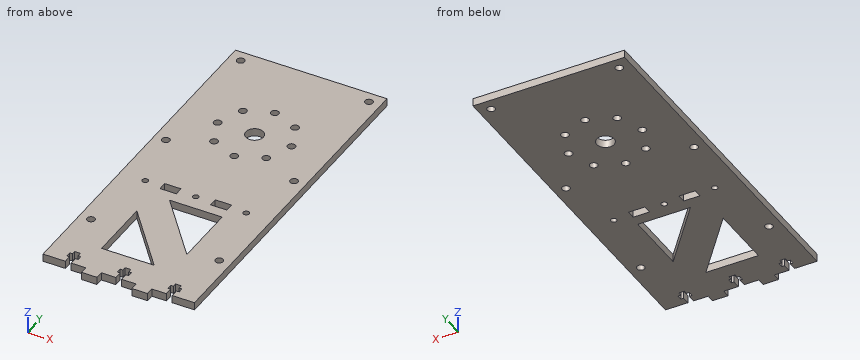
```python
from build123d import *

# Parameters (mm, degrees)
SKETCH_1_W          = 78
SKETCH_1_H          = 180
SKETCH_1_R          = 4.5
SKETCH_1_R_2        = 2
EXTRUDE_1_DEPTH     = 4
SKETCH_2_R          = 1.5
SKETCH_2_W          = 8.4
SKETCH_2_H          = 4.4
CUT_EXTRUDE_1_DEPTH = 4
SKETCH_6_W          = 8
SKETCH_6_H          = 8
EXTRUDE_2_DEPTH     = 4
SKETCH_7_R          = 2
CUT_EXTRUDE_2_DEPTH = 10


with BuildPart() as part:
    # 草图1 → 凸台-拉伸1 (new body)
    with BuildSketch(Plane.XY):
        with Locations((-4, -57.5)):
            Rectangle(SKETCH_1_W, SKETCH_1_H)
        with Locations((-4, -20.5)):
            Circle(SKETCH_1_R, mode=Mode.SUBTRACT)
        with Locations((15, -20.5)):
            Circle(SKETCH_1_R_2, mode=Mode.SUBTRACT)
        with Locations((9.435028843, -33.935028843)):
            Circle(SKETCH_1_R_2, mode=Mode.SUBTRACT)
        with Locations((-4, -39.5)):
            Circle(SKETCH_1_R_2, mode=Mode.SUBTRACT)
        with Locations((-17.435028843, -33.935028843)):
            Circle(SKETCH_1_R_2, mode=Mode.SUBTRACT)
        with Locations((-23, -20.5)):
            Circle(SKETCH_1_R_2, mode=Mode.SUBTRACT)
        with Locations((-17.435028843, -7.064971157)):
            Circle(SKETCH_1_R_2, mode=Mode.SUBTRACT)
        with Locations((-4, -1.5)):
            Circle(SKETCH_1_R_2, mode=Mode.SUBTRACT)
        with Locations((9.435028843, -7.064971157)):
            Circle(SKETCH_1_R_2, mode=Mode.SUBTRACT)
    extrude(amount=EXTRUDE_1_DEPTH)

    # 草图2 → 切除-拉伸1 (cut)
    with BuildSketch(Plane.XY.offset(4)):
        with Locations((-4, -75.5)):
            Circle(SKETCH_2_R)
        with Locations((22, -75.5)):
            Circle(SKETCH_2_R)
        with Locations((-30, -75.5)):
            Circle(SKETCH_2_R)
        with Locations((-17, -75.5)):
            Rectangle(SKETCH_2_W, SKETCH_2_H)
        with Locations((9, -75.5)):
            Rectangle(SKETCH_2_W, SKETCH_2_H)
        Polygon((-31.5, -147.5), (-31.5, -143.5), (-32.9, -143.5), (-32.9, -140.9), (-31.5, -140.9), (-31.5, -138.9), (-28.5, -138.9), (-28.5, -140.9), (-27.1, -140.9), (-27.1, -143.5), (-28.5, -143.5), (-28.5, -147.5), align=None)
        Polygon((23.5, -147.5), (20.5, -147.5), (20.5, -143.5), (19.1, -143.5), (19.1, -140.9), (20.5, -140.9), (20.5, -138.9), (23.5, -138.9), (23.5, -140.9), (24.9, -140.9), (24.9, -143.5), (23.5, -143.5), align=None)
        Polygon((-5.5, -147.5), (-5.5, -143.5), (-6.9, -143.5), (-6.9, -140.9), (-5.5, -140.9), (-5.5, -138.9), (-2.5, -138.9), (-2.5, -140.9), (-1.1, -140.9), (-1.1, -143.5), (-2.5, -143.5), (-2.5, -147.5), align=None)
    extrude(amount=-CUT_EXTRUDE_1_DEPTH, mode=Mode.SUBTRACT)

    # 草图6 → 凸台-拉伸2 (add)
    with BuildSketch(Plane.XY.offset(4)):
        with Locations((-17, -147.5)):
            Rectangle(SKETCH_6_W, SKETCH_6_H)
        with Locations((9, -147.5)):
            Rectangle(SKETCH_6_W, SKETCH_6_H)
    extrude(amount=-EXTRUDE_2_DEPTH)

    # 草图7 → 切除-拉伸2 (cut)
    with BuildSketch(Plane(origin=(0, 0, 0), x_dir=(-1, 0, 0), z_dir=(0, 0, -1))):
        with Locations((-29, 26.5)):
            Circle(SKETCH_7_R)
        with Locations((-29, -43.5)):
            Circle(SKETCH_7_R)
        with Locations((-29, -113.5)):
            Circle(SKETCH_7_R)
        with Locations((37, -43.5)):
            Circle(SKETCH_7_R)
        with Locations((37, -113.5)):
            Circle(SKETCH_7_R)
        with Locations((37, 26.5)):
            Circle(SKETCH_7_R)
        Polygon((-14, -83.5), (-14, -116.531181995), (13.091821195, -83.5), align=None)
        Polygon((-5.091821195, -130.9), (22, -97.868818005), (22, -130.9), align=None)
    extrude(amount=-CUT_EXTRUDE_2_DEPTH, mode=Mode.SUBTRACT)


solid = part.part
```
The model under review builds one solid part; all positions refer to its coordinate system, in mm. Round coordinates to 2 decimals unless told otherwise and drop trailing zeros. Write each loop counter-clockwise with the first axis right and the second up, starting at its lowest first coordinate (ties: lowest second). Pieces come first, ordered by that corner, then holes. Notation, with made-up numbers: (33, -33) - (40, -33) arc R9 cw to (40, -19) - close; hole circle Ø10 at (70.25, 57). An arc over 180 degrees is marked (long way). Use one line per item in the form item = value.
Q1. Consider section D-D (z = 1.7). State how many separate pieces and enclosed holes the cut face has, and give its area (3 significant figures).
Answer key:
separate_pieces = 1
enclosed_holes = 22
area = 12,800 mm2
Q2. For line 1 (Y direction, x = -37, z = 1.75); line 2 (X direction, y = -19, z = 2.1); line 3 (Y direction, x = 4, z = 1.25), list the stretches that pass through material, from the lowest coordinate up. Write a range as [from, to].
Answer key:
line_1 = [-147.5, -115.5], [-111.5, -45.5], [-41.5, 24.5], [28.5, 32.5]
line_2 = [-43, -24.32], [-21.68, -8.24], [0.24, 13.68], [16.32, 35]
line_3 = [-147.5, -130.9], [-129.57, -104.34], [-83.5, 32.5]
Q3. Consider section A-A (y = -20.5). State the section outline as (x, z) points, and give its area (3 significant figures).
Answer key:
outline = (-43, 0) - (-25, 0) - (-25, 4) - (-43, 4) - close; (-21, 0) - (-8.5, 0) - (-8.5, 4) - (-21, 4) - close; (0.5, 0) - (13, 0) - (13, 4) - (0.5, 4) - close; (17, 0) - (35, 0) - (35, 4) - (17, 4) - close
area = 244 mm2
Q4. Consider section B-B (x = 29). State the section outline as (y, z) points, and give its area (3 significant figures).
Answer key:
outline = (-147.5, 0) - (-115.5, 0) - (-115.5, 4) - (-147.5, 4) - close; (-111.5, 0) - (-45.5, 0) - (-45.5, 4) - (-111.5, 4) - close; (-41.5, 0) - (24.5, 0) - (24.5, 4) - (-41.5, 4) - close; (28.5, 0) - (32.5, 0) - (32.5, 4) - (28.5, 4) - close
area = 672 mm2
Q5. Consider section C-C (y = -43.5). State the section outline as (x, z) points.
Answer key:
outline = (-43, 0) - (-39, 0) - (-39, 4) - (-43, 4) - close; (-35, 0) - (27, 0) - (27, 4) - (-35, 4) - close; (31, 0) - (35, 0) - (35, 4) - (31, 4) - close
Q6. Insertion check: pin 1 Ø6.5 at (x, y) = (-37, -113.5) entering from -Z; pin 2 Ø1.2 at (x, z) = (-9, 1) entering from -Y. Each pin has a flat end and moves straight along its axis. Give the tip position at first contact, or say it passes through.
Answer key:
pin_1 = 0
pin_2 = -147.5
